Input: part model. Units: mm. Frame: model coordinates. Face numbers are marked on the shaded views. A direction names the side the tool comes from. Coordinates: 2 decimals unless noted, no trailing zeros. Order: outer loops, then holes, each group sorted by start corner. A loop starts at its lowest first (then second) coordinate and runs counter-clockwise, first axis right, second up. Notation, with made-up numbers: (-36.75, 8) - (-1.75, 8) arc R30 ccw to (-1.75, 45) - close; hole circle Ø8 at (84.5, 88.25). An arc over 180 degrees is marked (long way). Answer as CSV lines item,"result". Start each with the question number.
Item 1: Section B-B (x = 65). Output: boundary loops of the cut face in (y, z).
Item 2: Material intervals for line 1 along X through (y, z) = (5.25, -4); line 2 along Y through (x, z) = (51, -1.5); line 3 along X through (y, z) = (-4, -5.5), sorted ascending.
Item 3: First-contact query: pin 1 (2.5 mm diameter, centred on x = 48.5, z = -0.5, fed in from +Y); pin 2 (4.5 mm diameter, centred on x = 64.5, z = -2, fed in from -Y); pin 3 (5 mm diameter, centred on x = 44.5, y = -0.5, fed in from +Z); pin 4 (5 mm diameter, centred on x = -51, y = 0.5, fed in from -Z). Flat tips, straight axial feed; report the tip coordinate or a pass-through.
Item 4: Draft query along X for the marked faces 1, 2, 3 and 4. Return one class per face: +X half, -X half, draft (parallel to the pull), parting line (faces both ways), or undercut.
Item 5: Section C-C (x = -26.5). Output: boundary loops of the cut face in (y, z), and give its area (3 significant figures).
Item 6: Access query for the marked faces 5, 6 and 7. Directions: +Z, -Z, +X, -X, +Y, -Y. A direction counts if a zero-diameter tool reaches every point of the face in a straight line with its end or side. Return the directions, or none.
Item 7: Section A-A (z = 0). Output: boundary loops of the cut face in (x, y).
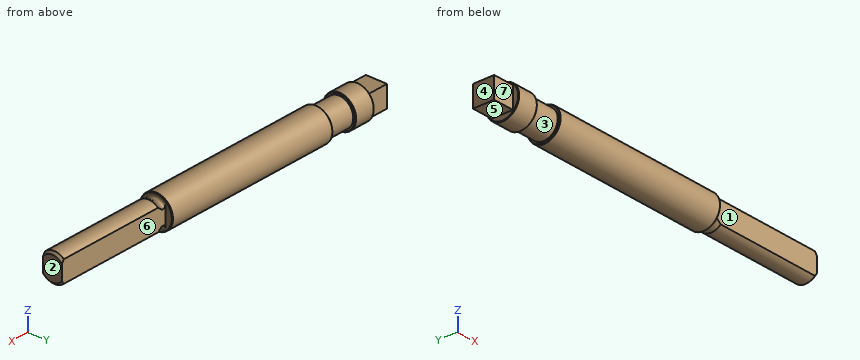
from build123d import *

# Parameters (mm, degrees)
SCHNITT_LINEAR_AUSTRAGEN1_DEPTH      = 87.078562226
SCHNITT_LINEAR_AUSTRAGEN1_DEPTH_BACK = 87.078562226
SKIZZE4_W                            = 136.51116069
SKIZZE4_H                            = 4.996766738
SCHNITT_LINEAR_START                 = -9
SKIZZE5_R                            = 7
SKIZZE5_W                            = 9
SKIZZE5_H                            = 9
SCHNITT_LINEAR_AUSTRAGEN2_DEPTH      = 9
FASE1_SIZE                           = 0.25


# Read off the part's stored shape, not the designer's step: M12 Maschinengewinde Bolzen1
with BuildPart() as part:
    # Skizze2 → Rotation1 (revolve)
    with BuildSketch(Plane.XY, mode=Mode.PRIVATE) as rotation1_sk:
        Polygon((35.507419999, 7), (35.507419999, 6), (85.507419999, 6), (85.507419999, 0), (-70.992580001, 0), (-70.992580001, 7), (-52.992580001, 7), (-52.992580001, 6), (-41.992580001, 6), (-41.992580001, 7), align=None)
    revolve(rotation1_sk.sketch.rotate(Axis((-31.289719626, 0, 0), (1, 0, 0)), 90), axis=Axis((-31.289719626, 0, 0), (1, 0, 0)))

    # M12 Maschinengewinde Bolzen1 outline → M12 Maschinengewinde Bolzen1 (revolve, cut)
    with BuildSketch(Plane.YX):
        with BuildLine():
            Line((6, 39.007419999), (5.133974596, 37.507419999))
            ThreePointArc((5.133974596, 37.507419999), (5.034074174, 37.266239044), (5, 37.007419999))
            Line((5, 37.007419999), (5, 36.507419999))
            ThreePointArc((5, 36.507419999), (5.292893219, 35.800313218), (6, 35.507419999))
            Line((6, 35.507419999), (6, 39.007419999))
        make_face()
        Polygon((5.036, 85.507419999), (6, 84.543419999), (6, 85.507419999), align=None)
    revolve(axis=Axis((0, 0, 0), (1, 0, 0)), mode=Mode.SUBTRACT)

    # Skizze4 → Schnitt-Linear austragen1 (cut, two sides: drawn at the far end of the back side and taken through both)
    with BuildSketch(Plane.XY.offset(-SCHNITT_LINEAR_AUSTRAGEN1_DEPTH_BACK)):
        with Locations((103.763000344, 6.498383369)):
            Rectangle(SKIZZE4_W, SKIZZE4_H)
        with Locations((103.763000344, -6.498383369)):
            Rectangle(SKIZZE4_W, SKIZZE4_H)
    extrude(amount=SCHNITT_LINEAR_AUSTRAGEN1_DEPTH + SCHNITT_LINEAR_AUSTRAGEN1_DEPTH_BACK, mode=Mode.SUBTRACT)

    # Skizze5 → Schnitt-Linear austragen2 (cut)
    with BuildSketch(Plane.ZY.offset(70.992580001).offset(SCHNITT_LINEAR_START)):
        Circle(SKIZZE5_R)
        Rectangle(SKIZZE5_W, SKIZZE5_H, mode=Mode.SUBTRACT)
    extrude(amount=SCHNITT_LINEAR_AUSTRAGEN2_DEPTH, mode=Mode.SUBTRACT)

    # Fase1
    fase1_edges = [part.edges().sort_by_distance(p)[0] for p in [
        (-61.992580001, 0, -7),
        (-41.992580001, 0, -7),
        (-52.992580001, 0, -7),
        (35.507419999, 0, -7),
    ]]
    chamfer(fase1_edges, length=FASE1_SIZE)


solid = part.part
Determined:
1,outline,"(-4, -4.47) arc R6 ccw to (4, -4.47) - (4, 4.47) arc R6 ccw to (-4, 4.47) - close"
2,line 1,"x = -61.99 to -52.99, -41.99 to 35.51"
2,line 2,"y = -4 to 4"
2,line 3,"x = -61.94 to -53.04, -41.94 to 35.46"
3,pin 1,"stops at y = 4"
3,pin 2,"stops at y = -4"
3,pin 3,"stops at z = 6"
3,pin 4,"stops at z = -7"
4,face 1,"draft"
4,face 2,"+X half"
4,face 3,"undercut"
4,face 4,"-X half"
5,outline,"circle Ø14 at (0, 0)"
5,area,"154 mm^2"
6,face 5,"-Z, -X, +Y, -Y"
6,face 6,"+Z, -Z, +X, +Y"
6,face 7,"+Z, -Z, -X, -Y"
7,outline,"(-70.99, -4.5) - (-61.99, -4.5) - (-61.99, -6.75) - (-61.74, -7) - (-53.24, -7) - (-52.99, -6.75) - (-52.99, -6) - (-41.99, -6) - (-41.99, -6.75) - (-41.74, -7) - (35.26, -7) - (35.51, -6.75) - (35.51, -4) - (85.51, -4) - (85.51, 4) - (35.51, 4) - (35.51, 6.75) - (35.26, 7) - (-41.74, 7) - (-41.99, 6.75) - (-41.99, 6) - (-52.99, 6) - (-52.99, 6.75) - (-53.24, 7) - (-61.74, 7) - (-61.99, 6.75) - (-61.99, 4.5) - (-70.99, 4.5) - close"
